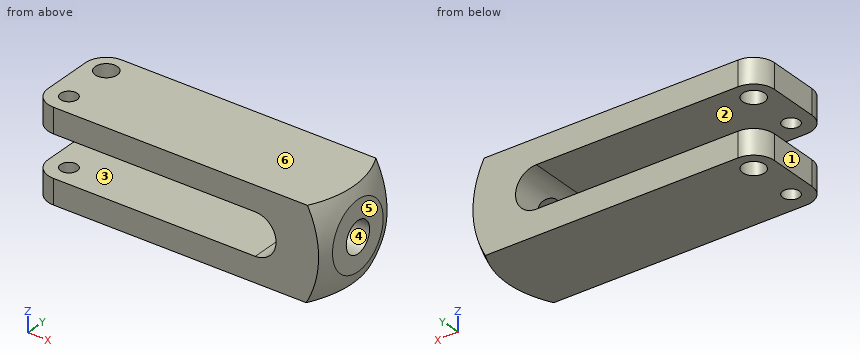
from build123d import *

# Parameters (mm, degrees)
F0_W     = 111.125
F0_H     = 34.925
F1_DEPTH = 34.925
F3_DEPTH = 34.925
F8_D     = 8.4328
F9_D     = 6.35
F10_R    = 7.9375
F12_D    = 11.90498


with BuildPart() as f1:
    # F0 (on Front) → F1 (new body)
    with BuildSketch(Plane.XZ):
        with Locations((-1.9895918667, -10.3187973859)):
            Rectangle(F0_W, F0_H)
    extrude(amount=F1_DEPTH)

    # F2 (on face) → F3 (cut)
    with BuildSketch(Plane.XZ.offset(34.925)):
        with BuildLine():
            Line((27.4617081333, -2.3812973859), (-57.5520918667, -2.3812973859))
            Line((-57.5520918667, -2.3812973859), (-57.5520918667, -18.2562973859))
            Line((-57.5520918667, -18.2562973859), (27.4617081333, -18.2562973859))
            ThreePointArc((27.4617081333, -18.2562973859), (35.3992081333, -10.3187973859), (27.4617081333, -2.3812973859))
        make_face()
    extrude(amount=-F3_DEPTH, mode=Mode.SUBTRACT)

    # F5 (on mid) → F6 (revolve, intersect)
    with BuildSketch(Plane.XZ.offset(17.4625)):
        with BuildLine():
            Line((-68.8055506017, -9.8742973859), (56.133069098, -9.8742973859))
            ThreePointArc((56.133069098, -9.8742973859), (52.8530157752, 4.9131087603), (44.7397269309, 17.70375669))
            Line((44.7397269309, 17.70375669), (-68.8055506017, 17.70375669))
            Line((-68.8055506017, 17.70375669), (-68.8055506017, -9.8742973859))
        make_face()
    revolve(axis=Axis((-6.3362407519, -17.4625, -9.8742973859), (-1, 0, 0)), mode=Mode.INTERSECT)

    # F8 (through all)
    with Locations(Plane.XY.offset(7.1437026141)):
        with Locations((-49.6145918667, -7.9375)):
            Hole(F8_D / 2)

    # F9 (through all)
    with Locations(Plane.XY.offset(7.1437026141)):
        with Locations((-49.6145918667, -26.9875)):
            Hole(F9_D / 2)

    # F10
    f10_edges = [f1.edges().sort_by_distance(p)[0] for p in [
        (-57.552092, 0, 2.381203),
        (-57.552092, -34.925, 2.381203),
        (-57.552092, 0, -23.018797),
        (-57.552092, -34.925, -23.018797),
    ]]
    fillet(f10_edges, radius=F10_R)

    # F12 (through all)
    with Locations(Plane.YZ.offset(53.5729081333)):
        with Locations((-17.4315758049, -10.4321427643)):
            Hole(F12_D / 2)


solid = f1.part
Source: CAD feature listing. Evaluate the final solid. Frame: model axes, mm. Face numbers are marked on the shaded views. A direction names the side the tool comes from. Coordinates: 2 decimals unless noted, no trailing zeros. Loops run counter-clockwise (first coordinate to the right, second up) from the corner with the lowest first, then second, coordinate; pieces in that order, holes last. Notation, with made-up numbers: (-19, -9) - (28, -9) arc R12 cw to (28, 0) - close; hole circle Ø3 at (39, 31). An arc over 180 degrees is marked (long way). One line per item, written item: value. Start each with the question number.
1. Section A-A (x = 2). Return the cut outline in (y, z) (3 decimals), and give its area (3 significant figures).
2. Section B-B (x = 31). Return the cut outline in (y, z) (3 decimals).
3. Ray query, L1, parallel to Z at x = -42, y = -8; L2, parallel to X at y = -28, z = -10.5; L3, parallel to Y at x = -48, z = 5.5 (3 decimals). Return the intervals inside material, ascending.
4. Section C-C (z = -21). State how many separate pieces and enclosed holes the cut face has, and give its area (3 significant figures).
5. Set-up query: the marked faces 1 and 2. Return all of +Z, -Z, +X, -X, +Y, -Y with unobstructed straight access to the full face (end or side cutting, diameter ignored); none if empty.
6. Contact query for flat-ended pins moving along their axis: P1, Ø10, axis at x = 23.5, z = -15.5, coming from the -Y side (3 decimals); P2, Ø6.5, axis at x = -49.61, y = -7.94, coming from the +Z side. Output: stop coordinate, or through.
7. Mould query, pull axis Z, two halves, no side actions, for the marked faces 3, 4, 5 and 6. Classes: pulls with the +Z half, pulls with the -Z half, needs draft (parallel to the pull), parting line crosses it, or undercut.
Verdict:
1. outline: (-34.925, -27.781) - (0, -27.781) - (0, -18.256) - (-34.925, -18.256) - close; (-34.925, -2.381) - (0, -2.381) - (0, 7.144) - (-34.925, 7.144) - close
1. area: 665 mm2
2. outline: (-34.925, -27.781) - (0, -27.781) - (0, -17.424) - (-34.925, -17.424) - close; (-34.925, -3.214) - (0, -3.214) - (0, 7.144) - (-34.925, 7.144) - close
3. L1: z = -27.78 to -18.26, -2.38 to 7.14
3. L2: x = 35.4 to 53.57
3. L3: y = -34.925 to -29.721, -24.254 to -11.833, -4.042 to 0
4. separate pieces: 1
4. enclosed holes: 2
4. area: 3,730 mm2
5. face 1: +Z, -Z, -X, +Y, -Y
5. face 2: -X, +Y, -Y
6. P1: stops at y = -34.925
6. P2: passes through
7. face 3: undercut
7. face 4: undercut
7. face 5: needs draft
7. face 6: pulls with the +Z half
